```python
from build123d import *

# Parameters (mm, degrees)
CYLINDER007_R     = 5
CYLINDER007_DEPTH = 14
CYLINDER006_R     = 8.5
CYLINDER006_DEPTH = 14
BOX006_W          = 10
BOX006_H          = 13
BOX006_DEPTH      = 14


with BuildPart() as lock_cut_bottom001:
    # Cylinder007 → Cylinder007 (new body)
    with BuildSketch(Plane(origin=(0, -11, 0), x_dir=(1, 0, 0), z_dir=(0, 0, 1))):
        Circle(CYLINDER007_R)
    extrude(amount=CYLINDER007_DEPTH)


with BuildPart() as lock_cut_top001:
    # Cylinder006 → Cylinder006 (new body)
    with BuildSketch(Plane(origin=(0, 8, 0), x_dir=(1, 0, 0), z_dir=(0, 0, 1))):
        Circle(CYLINDER006_R)
    extrude(amount=CYLINDER006_DEPTH)


with BuildPart() as lock:
    # Box006 → Box006 (new body)
    with BuildSketch(Plane(origin=(-5, -11, 0), x_dir=(1, 0, 0), z_dir=(0, 0, 1))):
        with Locations((5, 6.5)):
            Rectangle(BOX006_W, BOX006_H)
    extrude(amount=BOX006_DEPTH)

    # Fusion004: union lock cut bottom001, lock cut top001
    add(lock_cut_bottom001.part)
    add(lock_cut_top001.part)


with BuildPart() as lock_1:
    # Fusion004 placement: moved
    add(lock.part.moved(Location((0, -8, 0))))


solid = lock_1.part
```
Design review of the part built by this model. Coordinates are the model's own, in mm. A direction names the side the tool comes from. Round coordinates to 2 decimals unless told otherwise and drop trailing zeros. Write each loop counter-clockwise with the first axis right and the second up, starting at its lowest first coordinate (ties: lowest second). Pieces come first, ordered by that corner, then holes. Notation, with made-up numbers: (41.5, 27.5) -> (99.5, 27.5) arc R28 cw to (99.5, 53.5) -> close; hole circle Ø7 at (89, -28). An arc over 180 degrees is marked (long way). Write item = value, one per line. Start each with the question number.
1) Take a section at A-A, the plane y = -8. State the section outline as (x, z) points, plus the area to 3 significant figures.
2) Wall thickness on probe 1 along X at (y, z) = (-7, 3.25); probe 2 along Y at (x, z) = (-0.25, 9.75); probe 3 along Y at (x, z) = (-7.5, 13.25): over which ranges is each line inside the solid? List them lowest first. Write a range as from..to.
3) Take a section at B-B, the plane z = 8. State the section outline as (x, y) points, plus the area to 3 significant figures.
4) Clearance check with flat-ended pins moving along their axes: pin 1 (8 mm diameter, centred on y = -11.5, z = 3.5, fed in from -X); pin 2 (1.5 mm diameter, centred on x = -1.5, z = 6.5, fed in from +Y); pin 3 (3.5 mm diameter, centred on y = -15, z = 10.5, fed in from +X); pin 4 (1.5 mm diameter, centred on x = -5, y = -1, fed in from -Z). State where each tip first meets the part, or that it passes through.
5) Tool access review of faces 1 (the face through (0, -8, 0)), 2 (the face through (5, -13, 7)), 3 (the face through (-5, -13, 7)): name each direction out of +Z, -Z, +X, -X, +Y, -Y from which nothing blocks a thin tool from reaching the whole face with its end or side.
Results list:
q1.outline = (-5, 0) -> (5, 0) -> (5, 14) -> (-5, 14) -> close
q1.area = 140 mm²
q2.probe_1 = -5..5
q2.probe_2 = -23.99..8.5
q2.probe_3 = -4..4
q3.outline = (-5, -19) arc R5 ccw to (5, -19) -> (5, -6.87) arc R8.5 ccw (long way) to (-5, -6.87) -> close
q3.area = 376 mm²
q4.pin_1 = -5
q4.pin_2 = 8.47
q4.pin_3 = 5
q4.pin_4 = 0
q5.face_1 = -Z, +X, -X, +Y, -Y
q5.face_2 = +Z, -Z, +X, -Y
q5.face_3 = +Z, -Z, -X, -Y
